```python
from build123d import *

# Parameters (mm, degrees)
SKETCH1_W           = 15
SKETCH1_H           = 15
BOSS_EXTRUDE1_DEPTH = 30
SKETCH2_RX          = 12.112533461
SKETCH2_RY          = 6.212800173
CUT_EXTRUDE3_DEPTH  = 30
SKETCH3_R           = 2
CUT_EXTRUDE4_DEPTH  = 30


with BuildPart() as part:
    # Sketch1 → Boss-Extrude1 (new body)
    with BuildSketch(Plane(origin=(0, 0, 0), x_dir=(1, 0, 0), z_dir=(0, 1, 0))):
        with Locations((-41.148219583, -26.628215269)):
            Rectangle(SKETCH1_W, SKETCH1_H)
    extrude(amount=BOSS_EXTRUDE1_DEPTH)

    # Sketch2 → Cut-Extrude3 (cut)
    with BuildSketch(Plane(origin=(0, 0, 0), x_dir=(-1, 0, 0), z_dir=(0, -1, 0))):
        with Locations(Location((41.252812179, -19.128215269), (0, 0, -90))):
            Ellipse(SKETCH2_RX, SKETCH2_RY)
    extrude(amount=-CUT_EXTRUDE3_DEPTH, mode=Mode.SUBTRACT)

    # Sketch3 → Cut-Extrude4 (cut)
    with BuildSketch(Plane.ZY.offset(48.648219583)):
        with Locations((22.639015202, 15.346006291)):
            Circle(SKETCH3_R)
    extrude(amount=-CUT_EXTRUDE4_DEPTH, mode=Mode.SUBTRACT)


solid = part.part
```
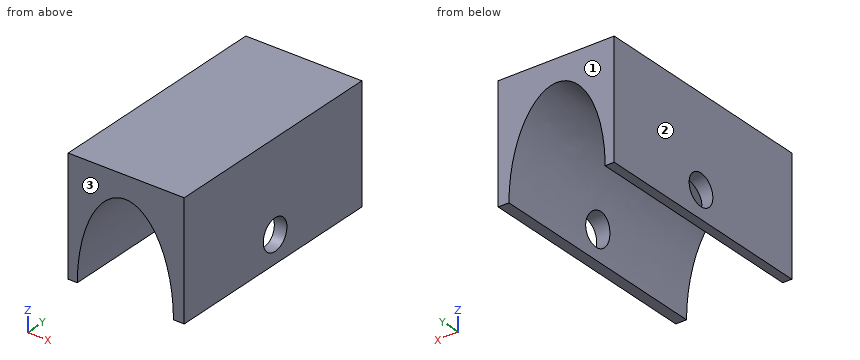
Geometry check sheet. Reference: the model listing, model coordinates, mm. Face numbers are marked on the shaded views. Round coordinates to 2 decimals unless told otherwise and drop trailing zeros. Order: outer loops, then holes, each group sorted by start corner. A loop starts at its lowest first (then second) coordinate and runs counter-clockwise, first axis right, second up. Notation, with made-up numbers: (43, 6.25) -> (59, 6.25) arc R16 cw to (59, 15.25) -> close; hole circle Ø3 at (84.5, 89). An arc over 180 degrees is marked (long way). Return JSON: item names as keys, results as strings. Group by question number.
Q1. Section check B-B, the plane z = 23.25. Count the separate pieces of the cut face and the enclosed holes in it, plus the area to 3 significant figures.
Q2. Material ranges on probe 1 along X at (y, z) = (11, 26); probe 2 along X at (y, z) = (8, 24); probe 3 along Z at (x, y) = (-36.5, 4.5), recorded low to high. Write a range as from..to.
Q3. Section check A-A, the plane x = -34.25. Record the boundary of the cut face in (y, z).
Q4. Release check for a two-part mould opening along Y. For the marked faces 1, 2 and 3 record: released by +Y, released by -Y, zero draft, split by the parting line, or undercut.
Numbers:
{
 "1": {"separate pieces": "4", "enclosed holes": "0", "area": "86.8 mm^2"},
 "2": {"probe 1": "-48.65..-46.37, -36.14..-33.65", "probe 2": "-48.65..-46.94, -35.56..-33.65", "probe 3": "26.93..34.13"},
 "3": {"outline": "(0, 19.13) -> (30, 19.13) -> (30, 34.13) -> (0, 34.13) -> close; hole circle Ø4 at (15.35, 22.64)"},
 "4": {"face 1": "released by +Y", "face 2": "zero draft", "face 3": "released by -Y"}
}
